Model file for the job. Use its own axes, mm. A direction names the side the tool comes from. Round coordinates to 2 decimals unless told otherwise and drop trailing zeros. Write each loop counter-clockwise with the first axis right and the second up, starting at its lowest first coordinate (ties: lowest second). Pieces come first, ordered by that corner, then holes. Notation, with made-up numbers: (55.5, 73.5) - (103.5, 73.5) arc R16 ccw to (103.5, 87.5) - close; hole circle Ø5 at (73.25, 13.5). An arc over 180 degrees is marked (long way). One line per item, written item: value.
from build123d import *

# Parameters (mm, degrees)
SKETCH3_R           = 12
BOSS_EXTRUDE1_DEPTH = 5
BOSS_EXTRUDE2_DEPTH = 5
SKETCH6_R           = 16
SKETCH6_R_2         = 12.5
SKETCH6_W           = 6
SKETCH6_H           = 6
CUT_EXTRUDE1_DEPTH  = 5


with BuildPart() as part:
    # Sketch3 → Boss-Extrude1 (new body)
    with BuildSketch(Plane.XY):
        Polygon((-77.781745931, 49.497474683), (-49.497474683, 77.781745931), (-43.840620434, 83.43860018), (43.840620434, 83.43860018), (49.497474683, 77.781745931), (77.781745931, 49.497474683), (88.388347648, 38.890872965), (27.497474683, -22), (-27.497474683, -22), (-88.388347648, 38.890872965), align=None)
        Circle(SKETCH3_R, mode=Mode.SUBTRACT)
        with Locations((0, 50)):
            Circle(SKETCH3_R, mode=Mode.SUBTRACT)
        Polygon((-81.317279836, 44.547727215), (-77.074639149, 48.790367902), (-72.831998462, 44.547727215), (-77.074639149, 40.305086528), align=None, mode=Mode.SUBTRACT)
        Polygon((-48.790367902, 77.074639149), (-44.547727215, 81.317279836), (-40.305086528, 77.074639149), (-44.547727215, 72.831998462), align=None, mode=Mode.SUBTRACT)
        Polygon((40.305086528, 77.074639149), (44.547727215, 72.831998462), (48.790367902, 77.074639149), (44.547727215, 81.317279836), align=None, mode=Mode.SUBTRACT)
        Polygon((72.831998462, 44.547727215), (77.074639149, 40.305086528), (81.317279836, 44.547727215), (77.074639149, 48.790367902), align=None, mode=Mode.SUBTRACT)
    extrude(amount=BOSS_EXTRUDE1_DEPTH)

    # Sketch5 → Boss-Extrude2 (add)
    with BuildSketch(Plane.XY.offset(5)):
        Polygon((-105.358910397, 38.890872965), (-49.811183182, 94.43860018), (49.811183182, 94.43860018), (105.358910397, 38.890872965), (29.468037432, -37), (-29.468037432, -37), align=None)
        Polygon((-43.840620434, 83.43860018), (-88.388347648, 38.890872965), (-27.497474683, -22), (27.497474683, -22), (88.388347648, 38.890872965), (43.840620434, 83.43860018), align=None, mode=Mode.SUBTRACT)
    extrude(amount=-BOSS_EXTRUDE2_DEPTH)

    # Sketch6 → Cut-Extrude1 (cut)
    with BuildSketch(Plane.XY.offset(5)):
        with Locations((-57, 58)):
            Circle(SKETCH6_R)
        with Locations((-57, 20)):
            Circle(SKETCH6_R_2)
        with Locations(Location((57, 20, 0), (0, 0, 180))):
            Circle(SKETCH6_R_2)
        with Locations(Location((57, 58, 0), (0, 0, 180))):
            Circle(SKETCH6_R)
        with Locations((-37, -19)):
            Rectangle(SKETCH6_W, SKETCH6_H)
        with Locations((37, -19)):
            Rectangle(SKETCH6_W, SKETCH6_H)
    extrude(amount=-CUT_EXTRUDE1_DEPTH, mode=Mode.SUBTRACT)


solid = part.part
1. Mould opens along Y. For faces 3 (the face through (40, -19, 3)), 4 (the face through (-66.88, 0.41, 2.54)), 5 (the face through (-1, 94.439, 3)) say: released by +Y, released by -Y, zero draft, split by the parting line, or undercut.
Report:
face 3: undercut
face 4: released by -Y
face 5: released by +Y
2. Band-saw the part on D-D on y = 22. Write the cut outline in (x, z), plus the area to 3 significant figures.
Report:
outline: (-88.47, 0) - (-69.34, 0) - (-69.34, 5) - (-88.47, 5) - close; (-44.66, 0) - (44.66, 0) - (44.66, 5) - (-44.66, 5) - close; (69.34, 0) - (88.47, 0) - (88.47, 5) - (69.34, 5) - close
area: 638 mm²
3. Tool access for faces 1 (the face through (42.46, 79.23, 2.46)), 2 (the face through (-77.97, 66.28, 2.54)): list every direction of +Z, -Z, +X, -X, +Y, -Y with a clear straight run to the whole face (end or side of a thin tool).
Report:
face 1: +Z, -Z
face 2: +Z, -Z, -X, +Y
4. Band-saw the part on B-B on y = 58. Write the cut outline in (x, z).
Report:
outline: (-86.25, 0) - (-73, 0) - (-73, 5) - (-86.25, 5) - close; (-41, 0) - (-8.94, 0) - (-8.94, 5) - (-41, 5) - close; (8.94, 0) - (41, 0) - (41, 5) - (8.94, 5) - close; (73, 0) - (86.25, 0) - (86.25, 5) - (73, 5) - close
5. Drop flat-ended pins along their axis: pin 1 (1.5 mm diameter, centred on y = -20, z = 3.5, fed in from +X); pin 2 (19 mm diameter, centred on x = 0, y = 50, fed in from +Z) (3 decimals); pin 3 (2 mm diameter, centred on x = -76, z = 4, fed in from -Y); pin 4 (1.5 mm diameter, centred on x = 36, z = 3, fed in from -Y). Give the stop position or say it passes through.
Report:
pin 1: x = 47.22
pin 2: through
pin 3: y = 8.53
pin 4: y = -31.22
6. Band-saw the part on A-A on x = 0. Write the cut outline in (y, z).
Report:
outline: (-37, 0) - (-12, 0) - (-12, 5) - (-37, 5) - close; (12, 0) - (38, 0) - (38, 5) - (12, 5) - close; (62, 0) - (94.44, 0) - (94.44, 5) - (62, 5) - close
7. Band-saw the part on C-C on z = 1.6. State how many separate pieces and enclosed holes the cut face has, plus the area to 3 significant figures.
Report:
separate pieces: 1
enclosed holes: 12
area: 15,100 mm²
8. Wall check: probe 1 along Y at (x, z) = (57, 3.15); probe 2 along Y at (x, z) = (-10, 1.45); probe 3 along X at (y, z) = (49.5, 3). Give the ranges that are in metal, low to high. Write a range as [from, to].
Report:
probe 1: [-9.47, 7.5], [32.5, 42], [74, 87.25]
probe 2: [-37, -6.63], [6.63, 43.37], [56.63, 94.44]
probe 3: [-94.75, -70.56], [-43.44, -11.99], [11.99, 43.44], [70.56, 94.75]
